Read the model definition and answer for the solid it produces. Units are mm, in the model's axes. A direction names the side the tool comes from. Coordinates: 2 decimals unless noted, no trailing zeros. Write each loop counter-clockwise with the first axis right and the second up, starting at its lowest first coordinate (ties: lowest second). Pieces come first, ordered by that corner, then holes.
(1) Which of the six approach directions +Z, -Z, +X, -X, +Y, -Y give full straight-line access (tool end or side, diameter ignored) to faces 5 (the cylindrical face through (1.32, -20.4, -0.57)), 6 (the cylindrical face through (-21.43, -10.4, -43.01)), 7 (the cylindrical face through (12.6, -22.01, -11.57))?
(2) Section B-B on y = 0 is taken. Write down the section's boundary in (x, z), then the cut area to 3 significant figures.
(3) Find the intervals of material crossed by probe 1 along Z at (x, y) = (-23, 15.5); probe 2 along Z at (x, y) = (-23.45, -15.5); probe 3 along Y at (x, z) = (16, 11.5), in increasing order.
(4) Given pin 1 (1.5 mm diameter, centred on x = 5, y = 3, fed in from -Z); pin 2 (2 mm diameter, centred on x = -6.5, z = -3, fed in from +Y); pin 3 (3 mm diameter, centred on y = 15.5, z = -36.5, fed in from +X); pin 4 (8 mm diameter, centred on y = -10, z = -31, fed in from +X), each flat-ended and moving along its own axis, determine where each tip first touches the part or whether it passes through.
(5) Section A-A on z = -21 is taken. Write down the section's boundary in (x, y).
(6) Section C-C on x = -15.5 is taken. Write down the section's boundary in (y, z).
(7) Section D-D on y = 15.5 is taken. Write down the section's boundary in (x, z), then the cut area to 3 significant figures.
(8) The mould has two halves that part along Y. Classify faces 1 (the cylindrical face through (-23.014, 15.934, -38.452)), 2 (the flat face through (0, -8.5, 14)), 3 (the cylindrical face through (-22.99, 20.43, -43.4)), 4 (the cylindrical face through (23.43, -22.01, -10.4)): +Y half, -Y half, draft (parallel to the pull), parting line (faces both ways), or undercut.
from build123d import *

# Parameters (mm, degrees)
SKETCH1_W                = 48
SKETCH1_H                = 29
BOSS_EXTRUDE1_DEPTH      = 29
SKETCH2_W                = 25
SKETCH2_H                = 25
CUT_EXTRUDE1_DEPTH       = 48
SKETCH3_W                = 48
SKETCH3_H                = 46
BOSS_EXTRUDE2_DEPTH      = 2
BOSS_EXTRUDE4_DEPTH      = 44
BOSS_EXTRUDE4_DEPTH_BACK = 2
SKETCH4_W                = 48
SKETCH4_H                = 2
SKETCH5_W                = 2
SKETCH5_H                = 46
BOSS_EXTRUDE5_DEPTH      = 44
SKETCH6_W                = 48
SKETCH6_H                = 12
BOSS_EXTRUDE6_DEPTH      = 2
SKETCH8_R                = 2
SKETCH8_R_2              = 12
CUT_EXTRUDE2_DEPTH       = 2
SKETCH9_W                = 12
SKETCH9_H                = 20
CUT_EXTRUDE3_DEPTH       = 2
FILLET4_R                = 2
SKETCH10_W               = 48
SKETCH10_H               = 10.5
BOSS_EXTRUDE7_DEPTH      = 29
SKETCH11_W               = 48
SKETCH11_H               = 2
CUT_EXTRUDE5_DEPTH       = 73
SKETCH13_W               = 25
SKETCH13_H               = 4
CUT_EXTRUDE6_DEPTH       = 73
SKETCH14_W               = 28
SKETCH14_H               = 14.5
BOSS_EXTRUDE10_DEPTH     = 48
FILLET5_R                = 2
FILLET6_R                = 2
FILLET7_R                = 2
FILLET8_R                = 2


with BuildPart() as part:
    # Sketch1 → Boss-Extrude1 (new body)
    with BuildSketch(Plane.XY):
        Rectangle(SKETCH1_W, SKETCH1_H)
    extrude(amount=BOSS_EXTRUDE1_DEPTH)

    # Sketch2 → Cut-Extrude1 (cut)
    with BuildSketch(Plane.ZY.offset(24)):
        with Locations((14.5, 0)):
            Rectangle(SKETCH2_W, SKETCH2_H)
    extrude(amount=-CUT_EXTRUDE1_DEPTH, mode=Mode.SUBTRACT)

    # Sketch3 → Boss-Extrude2 (add)
    with BuildSketch(Plane(origin=(0, 0, 0), x_dir=(-1, 0, 0), z_dir=(0, 0, -1))):
        Rectangle(SKETCH3_W, SKETCH3_H)
    extrude(amount=-BOSS_EXTRUDE2_DEPTH)

    # Sketch4 → Boss-Extrude4 (add, two sides: drawn at the far end of the back side and taken through both)
    with BuildSketch(Plane(origin=(0, 0, 0), x_dir=(-1, 0, 0), z_dir=(0, 0, -1)).offset(-BOSS_EXTRUDE4_DEPTH_BACK)):
        with Locations((0, -22)):
            Rectangle(SKETCH4_W, SKETCH4_H)
    extrude(amount=BOSS_EXTRUDE4_DEPTH + BOSS_EXTRUDE4_DEPTH_BACK)

    # Sketch5 → Boss-Extrude5 (add)
    with BuildSketch(Plane(origin=(0, 0, 0), x_dir=(-1, 0, 0), z_dir=(0, 0, -1))):
        with Locations((23, 0)):
            Rectangle(SKETCH5_W, SKETCH5_H)
    extrude(amount=BOSS_EXTRUDE5_DEPTH)

    # Sketch6 → Boss-Extrude6 (add)
    with BuildSketch(Plane(origin=(0, 0, -44), x_dir=(-1, 0, 0), z_dir=(0, 0, -1))):
        with Locations((0, -17)):
            Rectangle(SKETCH6_W, SKETCH6_H)
    extrude(amount=-BOSS_EXTRUDE6_DEPTH)

    # Sketch8 → Cut-Extrude2 (cut)
    with BuildSketch(Plane.ZY.offset(24)):
        with Locations(Location((-36.5, 15.5, 0), (0, 0, 270))):
            Circle(SKETCH8_R)
        with Locations(Location((-5.5, 15.5, 0), (0, 0, 270))):
            Circle(SKETCH8_R)
        with Locations(Location((-5.5, -15.5, 0), (0, 0, 270))):
            Circle(SKETCH8_R)
        with Locations(Location((-36.5, -15.5, 0), (0, 0, 270))):
            Circle(SKETCH8_R)
        with Locations(Location((-21, 0, 0), (0, 0, 270))):
            Circle(SKETCH8_R_2)
    extrude(amount=-CUT_EXTRUDE2_DEPTH, mode=Mode.SUBTRACT)

    # Sketch9 → Cut-Extrude3 (cut)
    with BuildSketch(Plane(origin=(0, -21, 0), x_dir=(1, 0, 0), z_dir=(0, 1, 0))):
        with Locations((18, 21)):
            Rectangle(SKETCH9_W, SKETCH9_H)
    extrude(amount=-CUT_EXTRUDE3_DEPTH, mode=Mode.SUBTRACT)

    # Fillet4
    fillet4_edges = [part.edges().sort_by_distance(p)[0] for p in [
        (-22, -11, -43),
    ]]
    fillet(fillet4_edges, radius=FILLET4_R)

    # Sketch10 → Boss-Extrude7 (add)
    with BuildSketch(Plane.XY.offset(29)):
        with Locations((0, 17.75)):
            Rectangle(SKETCH10_W, SKETCH10_H)
        with Locations((0, -17.75)):
            Rectangle(SKETCH10_W, SKETCH10_H)
    extrude(amount=-BOSS_EXTRUDE7_DEPTH)

    # Sketch11 → Cut-Extrude5 (cut)
    with BuildSketch(Plane.XY.offset(29)):
        with Locations((0, 22)):
            Rectangle(SKETCH11_W, SKETCH11_H)
    extrude(amount=-CUT_EXTRUDE5_DEPTH, mode=Mode.SUBTRACT)

    # Sketch13 → Cut-Extrude6 (cut)
    with BuildSketch(Plane.ZY.offset(24)):
        with Locations((14.5, 14.5)):
            Rectangle(SKETCH13_W, SKETCH13_H)
    extrude(amount=-CUT_EXTRUDE6_DEPTH, mode=Mode.SUBTRACT)

    # Sketch14 → Boss-Extrude10 (add)
    with BuildSketch(Plane.ZY.offset(24)):
        with Locations((15, -15.75)):
            Rectangle(SKETCH14_W, SKETCH14_H)
    extrude(amount=-BOSS_EXTRUDE10_DEPTH)

    # Fillet5
    fillet5_edges = [part.edges().sort_by_distance(p)[0] for p in [
        (1, -21, 0),
    ]]
    fillet(fillet5_edges, radius=FILLET5_R)

    # Fillet6
    fillet6_edges = [part.edges().sort_by_distance(p)[0] for p in [
        (1, -21, -42),
    ]]
    fillet(fillet6_edges, radius=FILLET6_R)

    # Fillet7
    fillet7_edges = [part.edges().sort_by_distance(p)[0] for p in [
        (-23, 21, -44),
    ]]
    fillet(fillet7_edges, radius=FILLET7_R)

    # Fillet8
    fillet8_edges = [part.edges().sort_by_distance(p)[0] for p in [
        (24, -22, -31),
        (24, -22, -11),
        (12, -22, -11),
        (12, -22, -31),
    ]]
    fillet(fillet8_edges, radius=FILLET8_R)


solid = part.part
Response:
1. face 5: +X, +Y
1. face 6: -Z, +X, +Y
1. face 7: +X, +Y, -Y
2. outline: (-24, -44) - (-22, -44) - (-22, -33) - (-24, -33) - close; (-24, -9) - (-22, -9) - (-22, 0) - (24, 0) - (24, 2) - (-24, 2) - close; (-24, 27) - (24, 27) - (24, 29) - (-24, 29) - close
2. area: 232 mm2
3. probe 1: z = -44 to -38.5, -34.5 to -7.5, -3.5 to 2, 27 to 29
3. probe 2: z = -44 to -38.5, -34.5 to -7.5, -3.5 to 29
3. probe 3: y = -23 to -8.5, 16.5 to 21
4. pin 1: stops at z = 0
4. pin 2: stops at y = -21
4. pin 3: passes through
4. pin 4: stops at x = -22
5. outline: (-24, -23) - (12, -23) - (12, -21) - (-22, -21) - (-22, -12) - (-24, -12) - close; (-24, 12) - (-22, 12) - (-22, 21) - (-24, 21) - close
6. outline: (-23, -44) - (-11, -44) - (-11, -42) - (-19, -42) arc R2 cw to (-21, -40) - (-21, -2) arc R2 cw to (-19, 0) - (21, 0) - (21, 29) - (-23, 29) - close; hole (-8.5, 2) - (16.5, 2) - (16.5, 27) - (-8.5, 27) - close
7. outline: (-24, -44) - (-22, -44) - (-22, -38.5) - (-24, -38.5) - close; (-24, -34.5) - (-22, -34.5) - (-22, -7.5) - (-24, -7.5) - close; (-24, -3.5) - (-22, -3.5) - (-22, 0) - (24, 0) - (24, 2) - (-24, 2) - close; (-24, 27) - (24, 27) - (24, 29) - (-24, 29) - close
7. area: 264 mm2
8. face 1: undercut
8. face 2: undercut
8. face 3: +Y half
8. face 4: draft
